Here's how the part is built. I have some questions about the finished solid (model axes, mm). Face numbers are marked on the shaded views. A direction names the side the tool comes from. Give positions to 0.01 mm unless a question says otherwise; leave off trailing zeros. Order: outer loops, then holes, each group sorted by start corner. A loop starts at its lowest first (then second) coordinate and runs counter-clockwise, first axis right, second up. Notation, with made-up numbers: M -31.75,46 L 25.25,46 A17 cw 25.25,61 Z; hole C -28.75,61 d3. An arc over 180 degrees is marked long. Use one line per item in the form item = value.
from build123d import *

# Parameters (mm, degrees)
SKETCH4_W          = 5.2
SKETCH4_H          = 3.2
CUT_EXTRUDE1_DEPTH = 4.3


with BuildPart() as part:
    # Sketch1 → Revolve2 (revolve)
    with BuildSketch(Plane.XY, mode=Mode.PRIVATE) as revolve2_sk:
        Polygon((0, 0), (2.5, 0), (1.893782217, 0.35), (100, 0.35), (100, 5.1), (0, 5.1), align=None)
    revolve(revolve2_sk.sketch.rotate(Axis((100, 5.1, 0), (-1, 0, 0)), 180), axis=Axis((100, 5.1, 0), (-1, 0, 0)))

    # Sketch4 → Cut-Extrude1 (cut)
    with BuildSketch(Plane(origin=(100, 0, 0), x_dir=(0, 0, -1), z_dir=(1, 0, 0))):
        with Locations((0, 5.1)):
            Rectangle(SKETCH4_W, SKETCH4_H)
    extrude(amount=-CUT_EXTRUDE1_DEPTH, mode=Mode.SUBTRACT)


solid = part.part
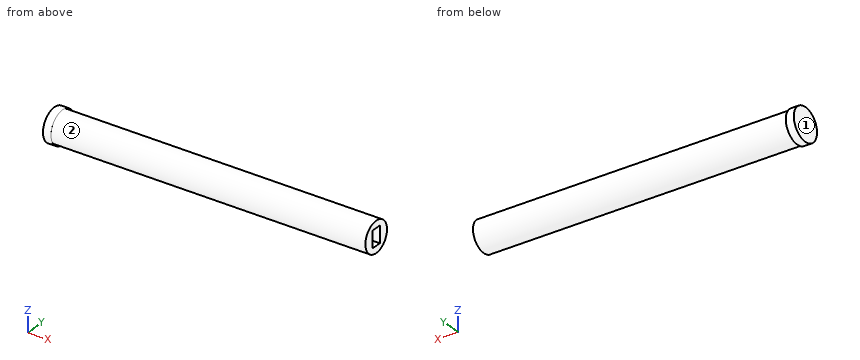
Q1. I need wall thicknesses on L1, parallel to X at y = 6.5, z = 1.5; L2, parallel to Z at x = 81, y = 5; L3, parallel to Y at x = 52, z = 3.25. Which ranges of each line are inside material? Lowest first, please.
Found:
L1 = 0 to 95.7
L2 = -4.75 to 4.75
L3 = 1.64 to 8.56
Q2. I'm going to push flat-ended pins straight in: pin 1 Ø3 at (x, z) = (44.5, 1) entering from -Y; pin 2 Ø1 at (x, z) = (30.5, 1) entering from +Y; pin 3 Ø1 at (x, y) = (98.5, 5.5) entering from +Z. Where does each tip first touch, or does it pass through?
Found:
pin_1 = 0.35
pin_2 = 9.82
pin_3 = 4.75
Q3. I want a section at A-A on z = 0. Write out the boundary of the cut face in (x, y), then the cut area to 3 significant figures.
Found:
outline = M 0,0 L 2.5,0 L 1.89,0.35 L 100,0.35 L 100,3.5 L 95.7,3.5 L 95.7,6.7 L 100,6.7 L 100,9.85 L 1.89,9.85 L 2.5,10.2 L 0,10.2 Z
area = 938 mm²
Q4. I want a section at B-B on y = 5.1. Write out the boundary of the cut face in (x, z), then the cut area to 3 significant figures.
Found:
outline = M 0,-5.1 L 2.5,-5.1 L 1.89,-4.75 L 100,-4.75 L 100,-2.6 L 95.7,-2.6 L 95.7,2.6 L 100,2.6 L 100,4.75 L 1.89,4.75 L 2.5,5.1 L 0,5.1 Z
area = 929 mm²
Q5. On a 3-axis mill with a long thin cutter (end or side, diameter ignored), from which of +Z, -Z, +X, -X, +Y, -Y can I reach the whole of each face in a straight line? I mean the marked faces 1 and 2. Say none if no direction works.
Found:
face_1 = +Z, -Z, -X, +Y, -Y
face_2 = +X
Q6. I want a section at C-C on x = 73. Write out the boundary of the cut face in (y, z).
Found:
outline = C 5.1,0 d9.5
